Work out the finished part from the listing and answer in its coordinate system (mm). A direction names the side the tool comes from. Round coordinates to 2 decimals unless told otherwise and drop trailing zeros. Use a Markdown table: item, result. Add a question column.
Item 1: A tool of negligible diameter and unlimited length cuts with its end or side. For faces 5 (the flat face through (-47, -292.99, 6)), 6 (the flat face through (147, 106.13, 6)), 7 (the flat face through (46, 292.99, 6)), 8 (the flat face through (127, 299, 6)), 9 (the flat face through (-147, -106.13, 6)), from which of +Z, -Z, +X, -X, +Y, -Y can it reach the whole face along a straight path? Write none if from no direction.
Item 2: For a pull along Y with two mould halves and no side action, classify faces 1 (the flat face through (-147, 80.73, 6)), 2 (the flat face through (-33.867, -299, 6)), 3 (the flat face through (140.59, 94, 6)), 4 (the flat face through (134, -292.99, 6)) as +Y half, -Y half, draft (parallel to the pull), parting line (faces both ways), or undercut.
Item 3: Find the intervals of material crossed by L1, parallel to X at y = -269, z = 3.25; L2, parallel to Y at x = 140, z = 11, in increasing order. Write a range as [from, to].
Item 4: Flat-ended cylindrical pins translate along their axes: P1, Ø2, axis at x = 58.5, z = 9, coming from the -Y side; P2, Ø3.5, axis at x = 146.5, z = 7.5, coming from the +Y side; P3, Ø3.5, axis at x = 148, z = 5, coming from the -Y side; P4, Ø6, axis at y = 274.5, z = 6, coming from the -X side. Find the tip coordinate at first contact, or state that the pin passes through.
from build123d import *

# Parameters (mm, degrees)
BASE_SKETCH_W           = 304.8
BASE_SKETCH_H           = 609.6
BOSS_EXTRUDE1_DEPTH     = 11.81
JOINT_X_W               = 25.4
JOINT_X_H               = 11.81
CUT_EXTRUDE1_DEPTH      = 341.981342745
LPATTERN1_COUNT         = 4
LPATTERN1_PITCH         = 93.133333333
MIRROR1_COPY_1_SKETCH_W = 25.4
MIRROR1_COPY_1_SKETCH_H = 11.81
MIRROR1_COPY_1_DEPTH    = 341.981342745
MIRROR1_COPY_2_SKETCH_W = 25.4
MIRROR1_COPY_2_SKETCH_H = 11.81
MIRROR1_COPY_2_DEPTH    = 341.981342745
MIRROR1_COPY_3_SKETCH_W = 25.4
MIRROR1_COPY_3_SKETCH_H = 11.81
MIRROR1_COPY_3_DEPTH    = 341.981342745
JOINT_Y_W               = 11.81
JOINT_Y_H               = 25.4
CUT_EXTRUDE2_DEPTH      = 341.981342745
LPATTERN3_COUNT         = 4
LPATTERN3_PITCH         = 186.86
MIRROR4_COPY_1_SKETCH_W = 11.81
MIRROR4_COPY_1_SKETCH_H = 25.4
MIRROR4_COPY_1_DEPTH    = 341.981342745
MIRROR4_COPY_2_SKETCH_W = 11.81
MIRROR4_COPY_2_SKETCH_H = 25.4
MIRROR4_COPY_2_DEPTH    = 341.981342745
MIRROR4_COPY_3_SKETCH_W = 11.81
MIRROR4_COPY_3_SKETCH_H = 25.4
MIRROR4_COPY_3_DEPTH    = 341.981342745


with BuildPart() as part:
    # Base_Sketch → Boss-Extrude1 (new body)
    with BuildSketch(Plane.XY):
        Rectangle(BASE_SKETCH_W, BASE_SKETCH_H)
    extrude(amount=BOSS_EXTRUDE1_DEPTH)

    # Joint_X → Cut-Extrude1 (cut, through all)
    with BuildSketch(Plane.XY.offset(11.81)):
        with Locations((-139.7, -298.895)):
            Rectangle(JOINT_X_W, JOINT_X_H)
    cut_extrude1 = extrude(amount=-CUT_EXTRUDE1_DEPTH, mode=Mode.SUBTRACT)

    # LPattern1: Cut-Extrude1 ×4
    with Locations(*[(i * LPATTERN1_PITCH, 0, 0) for i in range(1, LPATTERN1_COUNT)]):
        add(cut_extrude1, mode=Mode.SUBTRACT)

    # Mirror1: Cut-Extrude1 across plane
    add(cut_extrude1.mirror(Plane.ZX), mode=Mode.SUBTRACT)

    # Mirror1 copy 1 sketch → Mirror1 copy 1 (cut, through all)
    with BuildSketch(Plane(origin=(93.133333333, 0, 11.81), x_dir=(1, 0, 0), z_dir=(0, 0, 1))):
        with Locations((-139.7, 298.895)):
            Rectangle(MIRROR1_COPY_1_SKETCH_W, MIRROR1_COPY_1_SKETCH_H)
    extrude(amount=-MIRROR1_COPY_1_DEPTH, mode=Mode.SUBTRACT)

    # Mirror1 copy 2 sketch → Mirror1 copy 2 (cut, through all)
    with BuildSketch(Plane(origin=(186.266666667, 0, 11.81), x_dir=(1, 0, 0), z_dir=(0, 0, 1))):
        with Locations((-139.7, 298.895)):
            Rectangle(MIRROR1_COPY_2_SKETCH_W, MIRROR1_COPY_2_SKETCH_H)
    extrude(amount=-MIRROR1_COPY_2_DEPTH, mode=Mode.SUBTRACT)

    # Mirror1 copy 3 sketch → Mirror1 copy 3 (cut, through all)
    with BuildSketch(Plane(origin=(279.4, 0, 11.81), x_dir=(1, 0, 0), z_dir=(0, 0, 1))):
        with Locations((-139.7, 298.895)):
            Rectangle(MIRROR1_COPY_3_SKETCH_W, MIRROR1_COPY_3_SKETCH_H)
    extrude(amount=-MIRROR1_COPY_3_DEPTH, mode=Mode.SUBTRACT)

    # Joint_Y → Cut-Extrude2 (cut, through all)
    with BuildSketch(Plane.XY.offset(11.81)):
        with Locations((-146.495, -280.29)):
            Rectangle(JOINT_Y_W, JOINT_Y_H)
    cut_extrude2 = extrude(amount=-CUT_EXTRUDE2_DEPTH, mode=Mode.SUBTRACT)

    # LPattern3: Cut-Extrude2 ×4
    with Locations(*[(0, i * LPATTERN3_PITCH, 0) for i in range(1, LPATTERN3_COUNT)]):
        add(cut_extrude2, mode=Mode.SUBTRACT)

    # Mirror4: Cut-Extrude2 across plane
    add(cut_extrude2.mirror(Plane(origin=(0, 0, 0), x_dir=(0, 0, 1), z_dir=(1, 0, 0))), mode=Mode.SUBTRACT)

    # Mirror4 copy 1 sketch → Mirror4 copy 1 (cut, through all)
    with BuildSketch(Plane(origin=(0, 186.86, 11.81), x_dir=(-1, 0, 0), z_dir=(0, 0, 1))):
        with Locations((-146.495, 280.29)):
            Rectangle(MIRROR4_COPY_1_SKETCH_W, MIRROR4_COPY_1_SKETCH_H)
    extrude(amount=-MIRROR4_COPY_1_DEPTH, mode=Mode.SUBTRACT)

    # Mirror4 copy 2 sketch → Mirror4 copy 2 (cut, through all)
    with BuildSketch(Plane(origin=(0, 373.72, 11.81), x_dir=(-1, 0, 0), z_dir=(0, 0, 1))):
        with Locations((-146.495, 280.29)):
            Rectangle(MIRROR4_COPY_2_SKETCH_W, MIRROR4_COPY_2_SKETCH_H)
    extrude(amount=-MIRROR4_COPY_2_DEPTH, mode=Mode.SUBTRACT)

    # Mirror4 copy 3 sketch → Mirror4 copy 3 (cut, through all)
    with BuildSketch(Plane(origin=(0, 560.58, 11.81), x_dir=(-1, 0, 0), z_dir=(0, 0, 1))):
        with Locations((-146.495, 280.29)):
            Rectangle(MIRROR4_COPY_3_SKETCH_W, MIRROR4_COPY_3_SKETCH_H)
    extrude(amount=-MIRROR4_COPY_3_DEPTH, mode=Mode.SUBTRACT)


solid = part.part
Reported:
| question | item | result |
|---|---|---|
| 1 | face 5 | +Z, -Z, -Y |
| 1 | face 6 | +Z, -Z, +X |
| 1 | face 7 | +Z, -Z, +Y |
| 1 | face 8 | +Z, -Z, +X, +Y |
| 1 | face 9 | +Z, -Z, -X |
| 2 | face 1 | undercut |
| 2 | face 2 | draft |
| 2 | face 3 | undercut |
| 2 | face 4 | -Y half |
| 3 | L1 | [-140.59, 140.59] |
| 3 | L2 | [-292.99, 292.99] |
| 4 | P1 | y = -304.8 |
| 4 | P2 | y = 267.59 |
| 4 | P3 | y = -267.59 |
| 4 | P4 | x = -140.59 |
